Check sheet for the modelled part. Datum: model origin and axes. Units: mm. Face numbers are marked on the shaded views. Give positions to 0.01 mm unless a question says otherwise; leave off trailing zeros. Write each loop counter-clockwise with the first axis right and the second up, starting at its lowest first coordinate (ties: lowest second). Pieces come first, ordered by that corner, then holes. Notation, with made-up numbers: M 47.5,54 L 63.5,54 A25 ccw 63.5,73 Z; hole C -40,78.25 d3. An arc over 180 degrees is marked long. Use CSV: the item, a comma, the result in double quotes. Start each with the question number.
1. Cross-section at C-C, the plane z = 0. Enter the section's corners in (x, y), and give its area (3 significant figures).
2. Scan lines: line 1 (X direction, y = 55.5, z = 0); line 2 (X direction, y = 63.5, z = -2.25); line 3 (Y direction, x = -20, z = 3.25). Record each from-to range of solid material in increasing order.
3. Cross-section at A-A, the plane y = 61.5. Enter the section's corners in (x, z), and give its area (3 significant figures).
4. Depth check by flat-ended pin: P1, Ø2, axis at x = 14, z = 2, coming from the +Y side; P2, Ø3, axis at y = 32.5, z = 1.5, coming from the -X side; P3, Ø6, axis at x = -7.5, y = 76, coming from the +Z side. Enter the tip coordinate at first touch or a pass-through.
5. Cross-section at B-B, the plane x = 0. Enter the section's corners in (y, z).
6. Cross-section at D-D, the plane x = 14.5. Enter the section's corners in (y, z), and give its area (3 significant figures).
7. Mould release check, pull along Y, two halves, no side actions. Record for the marked faces 1, 2 and 3: +Y half, -Y half, draft (parallel to the pull), parting line (faces both ways), or undercut.
from build123d import *

# Parameters (mm, degrees)
SKETCH1_R            = 7
SKETCH1_R_2          = 4.75
SKETCH1_R_3          = 4
BOSS_EXTRUDE1_DEPTH  = 8
SKETCH1_3_R          = 4.75
SKETCH1_3_R_2        = 4
BOSS_EXTRUDE2_DEPTH  = 80
SKETCH3_R            = 5.75
SKETCH3_R_2          = 3.05
BOSS_EXTRUDE3_DEPTH  = 105
SKETCH8_W            = 50
SKETCH8_H            = 13
BOSS_EXTRUDE8_DEPTH  = 4
SKETCH9_W            = 50
SKETCH9_H            = 6.245985434
BOSS_EXTRUDE9_DEPTH  = 9
BOSS_EXTRUDE10_DEPTH = 50
SKETCH11_W           = 50
SKETCH11_H           = 12.98265639
BOSS_EXTRUDE11_DEPTH = 10
CUT_EXTRUDE1_DEPTH   = 100
SKETCH13_W           = 50
SKETCH13_H           = 13
BOSS_EXTRUDE12_DEPTH = 13
CUT_EXTRUDE2_DEPTH   = 50
CUT_EXTRUDE3_DEPTH   = 50


with BuildPart() as part:
    # Sketch1 → Boss-Extrude1 (new body)
    # profile 1 of 2: a face of its own
    with BuildSketch(Plane(origin=(0, 0, 0), x_dir=(1, 0, 0), z_dir=(0, 1, 0))):
        with Locations(Location((0, 0, 0), (0, 0, 270))):
            Circle(SKETCH1_R)
        Circle(SKETCH1_R_2, mode=Mode.SUBTRACT)
    # profile 2 of 2: a face of its own
    with BuildSketch(Plane(origin=(0, 0, 0), x_dir=(1, 0, 0), z_dir=(0, 1, 0))):
        Circle(SKETCH1_R_2)
        with Locations(Location((0, 0, 0), (0, 0, 270))):
            Circle(SKETCH1_R_3, mode=Mode.SUBTRACT)
    extrude(amount=BOSS_EXTRUDE1_DEPTH)

    # Sketch1_3 → Boss-Extrude2 (add)
    with BuildSketch(Plane(origin=(0, 0, 0), x_dir=(1, 0, 0), z_dir=(0, 1, 0))):
        with Locations(Location((0, 0, 0), (0, 0, 270))):
            Circle(SKETCH1_3_R)
        with Locations(Location((0, 0, 0), (0, 0, 270))):
            Circle(SKETCH1_3_R_2, mode=Mode.SUBTRACT)
    extrude(amount=BOSS_EXTRUDE2_DEPTH)

    # Sketch3 → Boss-Extrude3 (add)
    with BuildSketch(Plane.XZ):
        with Locations(Location((0, 0, 0), (0, 0, 270))):
            Circle(SKETCH3_R)
        with Locations(Location((0, 0, 0), (0, 0, 270))):
            Circle(SKETCH3_R_2, mode=Mode.SUBTRACT)
    extrude(amount=-BOSS_EXTRUDE3_DEPTH)

    # Sketch8 → Boss-Extrude8 (add)
    with BuildSketch(Plane(origin=(0, 105, 0), x_dir=(1, 0, 0), z_dir=(0, 1, 0))):
        Rectangle(SKETCH8_W, SKETCH8_H)
    extrude(amount=BOSS_EXTRUDE8_DEPTH)

    # Sketch9 → Boss-Extrude9 (add)
    with BuildSketch(Plane(origin=(0, 109, 0), x_dir=(1, 0, 0), z_dir=(0, 1, 0))):
        with Locations((0, -3.377007283)):
            Rectangle(SKETCH9_W, SKETCH9_H)
    extrude(amount=BOSS_EXTRUDE9_DEPTH)

    # Sketch10 → Boss-Extrude10 (add)
    with BuildSketch(Plane.ZY.offset(25)):
        with BuildLine():
            Line((0.254014566, 118), (0.254014566, 109))
            Line((0.254014566, 109), (-6.5, 109))
            ThreePointArc((-6.5, 109), (-4.986953748, 114.898802217), (0.254014566, 118))
        make_face()
    extrude(amount=-BOSS_EXTRUDE10_DEPTH)

    # Sketch11 → Boss-Extrude11 (add)
    with BuildSketch(Plane(origin=(0, 118, 0), x_dir=(1, 0, 0), z_dir=(0, 1, 0))):
        Rectangle(SKETCH11_W, SKETCH11_H)
    extrude(amount=-BOSS_EXTRUDE11_DEPTH)

    # Sketch12 → Cut-Extrude1 (cut)
    with BuildSketch(Plane(origin=(0, 0, -6.491328195), x_dir=(-1, 0, 0), z_dir=(0, 0, -1))):
        with BuildLine():
            Line((-25, 118), (25, 118))
            ThreePointArc((25, 118), (0, 116.124221553), (-25, 118))
        make_face()
    extrude(amount=-CUT_EXTRUDE1_DEPTH, mode=Mode.SUBTRACT)

    # Sketch13 → Boss-Extrude12 (add)
    with BuildSketch(Plane.XZ.offset(-105)):
        Rectangle(SKETCH13_W, SKETCH13_H)
    extrude(amount=-BOSS_EXTRUDE12_DEPTH)

    # Sketch14 → Cut-Extrude2 (cut)
    with BuildSketch(Plane.ZY.offset(25)):
        Polygon((-6.5, 105), (6.5, 118), (-6.5, 118), (-6.5, 107), align=None)
    extrude(amount=-CUT_EXTRUDE2_DEPTH, mode=Mode.SUBTRACT)


with BuildPart() as cut_extrude2_piece_1:
    # of the separate pieces the step leaves, piece 1, a body of its own (cut_extrude2_pieces)
    add(part.part.solids().sort_by_distance((-25, 105, -6.5))[0])


with BuildPart() as cut_extrude2_piece_2:
    # of the separate pieces the step leaves, piece 2, a body of its own (cut_extrude2_pieces)
    add(part.part.solids().sort_by_distance((-25, 109, -6.5))[0])

    # Sketch15 → Cut-Extrude3 (cut)
    with BuildSketch(Plane.ZY.offset(25)):
        with BuildLine():
            Line((6.5, 118), (-6.5, 105))
            Line((-6.5, 105), (-15.046764463, 116.293960334))
            Line((-15.046764463, 116.293960334), (5.81150646, 117.953140975))
            ThreePointArc((5.81150646, 117.953140975), (6.155619412, 117.978536655), (6.5, 118))
        make_face()
    extrude(amount=-CUT_EXTRUDE3_DEPTH, mode=Mode.SUBTRACT)


solid = cut_extrude2_piece_1.part
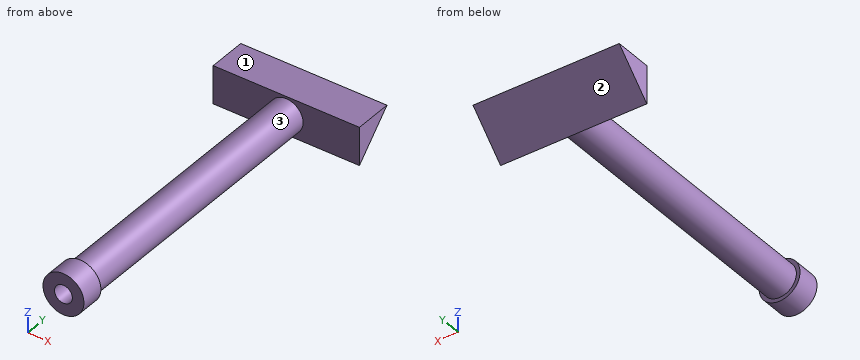
Worked answers:
1,outline,"M -25,105 L -5.75,105 L -5.75,8 L -7,8 L -7,0 L -3.05,0 L -3.05,105 L 3.05,105 L 3.05,0 L 7,0 L 7,8 L 5.75,8 L 5.75,105 L 25,105 L 25,111.5 L -25,111.5 Z"
1,area,"912 mm^2"
2,line 1,"x = -5.75 to -3.05, 3.05 to 5.75"
2,line 2,"x = -5.29 to -2.06, 2.06 to 5.29"
2,line 3,"y = 105 to 114.75"
3,outline,"C 0,0 d11.5; hole C 0,0 d6.1"
3,area,"74.6 mm^2"
4,P1,"stops at y = 114.5"
4,P2,"stops at x = -5.75"
4,P3,"stops at z = 3.58"
5,outline,"M 0,-7 L 8,-7 L 8,-5.75 L 105,-5.75 L 105,-6.5 L 118,6.5 L 105,6.5 L 105,5.75 L 8,5.75 L 8,7 L 0,7 L 0,3.05 L 105,3.05 L 105,-3.05 L 0,-3.05 Z"
6,outline,"M 105,-6.5 L 118,6.5 L 105,6.5 Z"
6,area,"84.5 mm^2"
7,face 1,"draft"
7,face 2,"+Y half"
7,face 3,"undercut"
